Verification items for the finished model (mm, model axes). A direction names the side the tool comes from. Give positions to 0.01 mm unless a question says otherwise; leave off trailing zeros. Write each loop counter-clockwise with the first axis right and the second up, starting at its lowest first coordinate (ties: lowest second). Pieces come first, ordered by that corner, then holes. Notation, with made-up numbers: M 37.5,44 L 81.5,44 A24 cw 81.5,56 Z; hole C 70.25,17.25 d3. An arc over 180 degrees is marked long. Answer as a JSON object with one key per item and string values.
```python
from build123d import *

# Parameters (mm, degrees)
CROQUIS4_R              = 9.7
SALIENTE_EXTRUIR2_DEPTH = 3.85
CROQUIS5_R              = 11.025
SALIENTE_EXTRUIR3_DEPTH = 2.1
CROQUIS6_R              = 9.65
SALIENTE_EXTRUIR4_DEPTH = 2.65
CROQUIS8_R              = 8.725
CORTAR_EXTRUIR2_DEPTH   = 4.05
CROQUIS9_R              = 2.35
CORTAR_EXTRUIR3_DEPTH   = 4.55
CROQUIS10_R             = 1.2
SALIENTE_EXTRUIR5_DEPTH = 4.05


with BuildPart() as part:
    # Croquis4 → Saliente-Extruir2 (new body)
    with BuildSketch(Plane(origin=(0, 0, 0), x_dir=(1, 0, 0), z_dir=(0, 1, 0))):
        with Locations(Location((0, 0, 0), (0, 0, 90))):
            Circle(CROQUIS4_R)
    extrude(amount=SALIENTE_EXTRUIR2_DEPTH)

    # Croquis5 → Saliente-Extruir3 (add)
    with BuildSketch(Plane(origin=(0, 3.85, 0), x_dir=(1, 0, 0), z_dir=(0, 1, 0))):
        with Locations(Location((0, 0, 0), (0, 0, 270))):
            Circle(CROQUIS5_R)
    extrude(amount=SALIENTE_EXTRUIR3_DEPTH)

    # Croquis6 → Saliente-Extruir4 (add)
    with BuildSketch(Plane(origin=(0, 5.95, 0), x_dir=(1, 0, 0), z_dir=(0, 1, 0))):
        with Locations(Location((0, 0, 0), (0, 0, 270))):
            Circle(CROQUIS6_R)
    extrude(amount=SALIENTE_EXTRUIR4_DEPTH)

    # Croquis8 → Cortar-Extruir2 (cut)
    with BuildSketch(Plane.XZ):
        with Locations(Location((0, 0, 0), (0, 0, 270))):
            Circle(CROQUIS8_R)
    extrude(amount=-CORTAR_EXTRUIR2_DEPTH, mode=Mode.SUBTRACT)

    # Croquis9 → Cortar-Extruir3 (cut)
    with BuildSketch(Plane(origin=(0, 8.6, 0), x_dir=(1, 0, 0), z_dir=(0, 1, 0))):
        with Locations(Location((-2.8, 4.849742261, 0), (0, 0, 270))):
            Circle(CROQUIS9_R)
        with Locations(Location((5.6, 0, 0), (0, 0, 270))):
            Circle(CROQUIS9_R)
        with Locations(Location((0, 0, 0), (0, 0, 270))):
            Circle(CROQUIS9_R)
        with Locations(Location((2.8, 4.849742261, 0), (0, 0, 270))):
            Circle(CROQUIS9_R)
        with Locations(Location((2.8, -4.849742261, 0), (0, 0, 270))):
            Circle(CROQUIS9_R)
        with Locations(Location((-2.800010296, -4.849760094, 0), (0, 0, 270))):
            Circle(CROQUIS9_R)
        with Locations(Location((-5.6, 0, 0), (0, 0, 270))):
            Circle(CROQUIS9_R)
    extrude(amount=-CORTAR_EXTRUIR3_DEPTH, mode=Mode.SUBTRACT)

    # Croquis10 → Saliente-Extruir5 (add)
    with BuildSketch(Plane.XZ.offset(-4.05)):
        with Locations((0, 8.3)):
            Circle(CROQUIS10_R)
        with Locations((-7.188010851, 4.15)):
            Circle(CROQUIS10_R)
        with Locations((-7.188010851, -4.15)):
            Circle(CROQUIS10_R)
        with Locations((0, -8.3)):
            Circle(CROQUIS10_R)
        with Locations((7.188010851, -4.15)):
            Circle(CROQUIS10_R)
        with Locations((7.188010851, 4.15)):
            Circle(CROQUIS10_R)
    extrude(amount=SALIENTE_EXTRUIR5_DEPTH)


solid = part.part
```
1) Go/stop test with flat-tipped pins: pin 1 (2 mm diameter, centred on x = 6.5, y = 4, fed in from -Z); pin 2 (3 mm diameter, centred on x = 5.5, z = 1.5, fed in from -Y); pin 3 (1.5 mm diameter, centred on y = 3, z = 2, fed in from +X). Record where each tip stops, or that it passes through.
Completed:
{"pin 1": "stops at z = -9.56", "pin 2": "stops at y = 4.05", "pin 3": "stops at x = 9.62"}
2) Section check C-C on z = -1. Record the boundary of the cut face in (x, y).
Completed:
{"outline": "M -10.98,3.85 L -9.65,3.85 L -9.65,0 L -8.67,0 L -8.67,4.05 L -7.73,4.05 L -7.73,8.6 L -9.6,8.6 L -9.6,5.95 L -10.98,5.95 Z; M -3.47,4.05 L -2.13,4.05 L -2.13,8.6 L -3.47,8.6 Z; M 2.13,4.05 L 3.47,4.05 L 3.47,8.6 L 2.13,8.6 Z; M 7.73,4.05 L 8.67,4.05 L 8.67,0 L 9.65,0 L 9.65,3.85 L 10.98,3.85 L 10.98,5.95 L 9.6,5.95 L 9.6,8.6 L 7.73,8.6 Z"}
3) Release check for a two-part mould opening along Z. For faces 1 (the face through (-2, 8.6, 2)), 2 (the face through (9.568, 7.256, -1.256)), 3 (the face through (6.165, 2.053, -3.523)) record: pulls with the +Z half, pulls with the -Z half, needs draft (parallel to the pull), parting line crosses it, or undercut.
Completed:
{"face 1": "needs draft", "face 2": "parting line crosses it", "face 3": "undercut"}
4) Section check A-A on x = 7.5. Record the boundary of the cut face in (y, z).
Completed:
{"outline": "M 0,-6.15 L 3.85,-6.15 L 3.85,-8.08 L 5.95,-8.08 L 5.95,-6.07 L 8.6,-6.07 L 8.6,-1.38 L 4.05,-1.38 L 4.05,-2.99 L 0,-2.99 Z; M 0,2.99 L 4.05,2.99 L 4.05,1.38 L 8.6,1.38 L 8.6,6.07 L 5.95,6.07 L 5.95,8.08 L 3.85,8.08 L 3.85,6.15 L 0,6.15 Z"}
5) Access from +Z, -Z, +X, -X, +Y, -Y to the whole of each face (thin tool, end or side, straight path). Record for faces 4 (the face through (-4.23, 6.357, 2.985)), 5 (the face through (-2, 4.05, -2)), 6 (the face through (-10, 5.95, 0)).
Completed:
{"face 4": "+Y, -Y", "face 5": "-Y", "face 6": "+Y"}
6) Thickness scan on L1, parallel to X at y = 5.85, z = 0 (3 decimals); L2, parallel to X at y = 7.05, z = 0; L3, parallel to Z at x = 1.25, y = 4.5. Record the ranges inside material, lowest first.
Completed:
{"L1": "x = -11.025 to -7.95, -3.25 to -2.35, 2.35 to 3.25, 7.95 to 11.025", "L2": "x = -9.65 to -7.95, -3.25 to -2.35, 2.35 to 3.25, 7.95 to 9.65", "L3": "z = -10.95 to -6.62, -3.08 to -1.99, 1.99 to 3.08, 6.62 to 10.95"}
7) Section check B-B on y = 1.75. Record the boundary of the cut face in (x, z) (3 decimals), and give its area (3 significant figures).
Completed:
{"outline": "C 0,0 d19.4; hole M -8.064,-3.33 A1.2 cw long -6.916,-5.319 A8.725 ccw -1.148,-8.649 A1.2 cw long 1.148,-8.649 A8.725 ccw 6.916,-5.319 A1.2 cw long 8.064,-3.33 A8.725 ccw 8.064,3.33 A1.2 cw long 6.916,5.319 A8.725 ccw 1.148,8.649 A1.2 cw long -1.148,8.649 A8.725 ccw -6.916,5.319 A1.2 cw long -8.064,3.33 A8.725 ccw Z", "area": "75.7 mm2"}
8) Section check D-D on y = 4.75. Record the boundary of the cut face in (x, z) (3 decimals).
Completed:
{"outline": "C 0,0 d22.05; hole C -5.6,0 d4.7; hole C -2.8,-4.85 d4.7; hole C -2.8,4.85 d4.7; hole C 0,0 d4.7; hole C 2.8,-4.85 d4.7; hole C 2.8,4.85 d4.7; hole C 5.6,0 d4.7"}
